```python
from build123d import *

# Parameters (mm, degrees)
SKETCH1_W                      = 229
SKETCH1_H                      = 200
BOSS_EXTRUDE1_DEPTH            = 1
CUT_EXTRUDE1_DEPTH             = 2
FILLET1_R                      = 8
FILLET2_R                      = 10
M3_CLEARANCE_HOLE1_AT_2_COUNT  = 2
M3_CLEARANCE_HOLE1_AT_2_PITCH  = 20
M3_CLEARANCE_HOLE1_AT_3_COUNT  = 2
M3_CLEARANCE_HOLE1_AT_3_PITCH  = 40
M3_CLEARANCE_HOLE1_AT_4_COUNT  = 2
M3_CLEARANCE_HOLE1_AT_4_PITCH  = 60
M3_CLEARANCE_HOLE1_AT_5_COUNT  = 2
M3_CLEARANCE_HOLE1_AT_5_PITCH  = 80
M3_CLEARANCE_HOLE1_AT_6_COUNT  = 2
M3_CLEARANCE_HOLE1_AT_6_PITCH  = 100
M3_CLEARANCE_HOLE1_AT_7_COUNT  = 2
M3_CLEARANCE_HOLE1_AT_7_PITCH  = 120
M3_CLEARANCE_HOLE1_AT_8_COUNT  = 2
M3_CLEARANCE_HOLE1_AT_8_PITCH  = 140
M3_CLEARANCE_HOLE1_AT_9_COUNT  = 2
M3_CLEARANCE_HOLE1_AT_9_PITCH  = 160
M3_CLEARANCE_HOLE1_AT_10_COUNT = 2
M3_CLEARANCE_HOLE1_AT_10_PITCH = 180
M3_CLEARANCE_HOLE2_AT_2_COUNT  = 2
M3_CLEARANCE_HOLE2_AT_2_PITCH  = 20
M3_CLEARANCE_HOLE2_AT_3_COUNT  = 2
M3_CLEARANCE_HOLE2_AT_3_PITCH  = 40
M3_CLEARANCE_HOLE2_AT_4_COUNT  = 2
M3_CLEARANCE_HOLE2_AT_4_PITCH  = 60
M3_CLEARANCE_HOLE2_AT_5_COUNT  = 2
M3_CLEARANCE_HOLE2_AT_5_PITCH  = 80
M3_CLEARANCE_HOLE2_AT_6_COUNT  = 2
M3_CLEARANCE_HOLE2_AT_6_PITCH  = 100
M3_CLEARANCE_HOLE2_AT_7_COUNT  = 2
M3_CLEARANCE_HOLE2_AT_7_PITCH  = 120
M3_CLEARANCE_HOLE2_AT_8_COUNT  = 2
M3_CLEARANCE_HOLE2_AT_8_PITCH  = 140
M3_CLEARANCE_HOLE2_AT_9_COUNT  = 2
M3_CLEARANCE_HOLE2_AT_9_PITCH  = 160
M3_CLEARANCE_HOLE2_AT_10_COUNT = 2
M3_CLEARANCE_HOLE2_AT_10_PITCH = 180
M3_CLEARANCE_HOLE2_AT_11_COUNT = 2
M3_CLEARANCE_HOLE2_AT_11_PITCH = 254.558441227
M3_CLEARANCE_HOLE2_AT_12_COUNT = 2
M3_CLEARANCE_HOLE2_AT_12_PITCH = 240.831891576
M3_CLEARANCE_HOLE2_AT_13_COUNT = 2
M3_CLEARANCE_HOLE2_AT_13_PITCH = 228.03508502
M3_CLEARANCE_HOLE2_AT_14_COUNT = 2
M3_CLEARANCE_HOLE2_AT_14_PITCH = 216.333076528
M3_CLEARANCE_HOLE2_AT_15_COUNT = 2
M3_CLEARANCE_HOLE2_AT_15_PITCH = 205.91260282
M3_CLEARANCE_HOLE2_AT_16_COUNT = 2
M3_CLEARANCE_HOLE2_AT_16_PITCH = 196.977156036
M3_CLEARANCE_HOLE2_AT_17_COUNT = 2
M3_CLEARANCE_HOLE2_AT_17_PITCH = 189.73665961
M3_CLEARANCE_HOLE2_AT_18_COUNT = 2
M3_CLEARANCE_HOLE2_AT_18_PITCH = 184.390889146
M3_CLEARANCE_HOLE2_AT_19_COUNT = 2
M3_CLEARANCE_HOLE2_AT_19_PITCH = 181.107702763
M3_CLEARANCE_HOLE2_AT_20_COUNT = 2
M3_CLEARANCE_HOLE2_AT_20_PITCH = 180
SKETCH7_R                      = 25
CUT_EXTRUDE2_DEPTH             = 10
FILLET3_R                      = 10
M4_CLEARANCE_HOLE1_AT_2_COUNT  = 2
M4_CLEARANCE_HOLE1_AT_2_PITCH  = 105
M4_CLEARANCE_HOLE1_AT_3_COUNT  = 2
M4_CLEARANCE_HOLE1_AT_3_PITCH  = 105
M4_CLEARANCE_HOLE1_AT_4_COUNT  = 2
M4_CLEARANCE_HOLE1_AT_4_PITCH  = 148.492424049
SKETCH10_R                     = 60
CUT_EXTRUDE3_DEPTH             = 10


with BuildPart() as part:
    # Sketch1 → Boss-Extrude1 (new body)
    with BuildSketch(Plane(origin=(0, 0, 0), x_dir=(1, 0, 0), z_dir=(0, 1, 0))):
        Rectangle(SKETCH1_W, SKETCH1_H)
    extrude(amount=BOSS_EXTRUDE1_DEPTH)

    # Sketch2 → Cut-Extrude1 (cut, through all)
    with BuildSketch(Plane(origin=(0, 1, 0), x_dir=(1, 0, 0), z_dir=(0, 1, 0))):
        Polygon((114.5, 60), (101.5, 73), (101.5, 100), (114.5, 100), align=None)
        Polygon((101.5, -100), (114.5, -100), (114.5, -60), (101.5, -73), align=None)
    extrude(amount=-CUT_EXTRUDE1_DEPTH, mode=Mode.SUBTRACT)

    # Fillet1
    fillet1_edges = [part.edges().sort_by_distance(p)[0] for p in [
        (114.5, 0.5, -60),
        (101.5, 0.5, -73),
        (101.5, 0.5, 73),
        (114.5, 0.5, 60),
    ]]
    fillet(fillet1_edges, radius=FILLET1_R)

    # Fillet2
    fillet2_edges = [part.edges().sort_by_distance(p)[0] for p in [
        (101.5, 0.5, -100),
        (101.5, 0.5, 100),
        (-114.5, 0.5, 100),
        (-114.5, 0.5, -100),
    ]]
    fillet(fillet2_edges, radius=FILLET2_R)

    # Sketch4 → M3 Clearance Hole1 (revolve, cut)
    with BuildSketch(Plane(origin=(-104.5, 0, -90), x_dir=(0, 0, -1), z_dir=(1, 0, 0))):
        Polygon((0, 0), (0, 1), (1.7, 1), (1.7, 0.025), (1.725, 0), align=None)
    m3_clearance_hole1 = revolve(axis=Axis((-104.5, -6.35, -90), (0, 1, 0)), mode=Mode.SUBTRACT)

    # M3 Clearance Hole1 at 2: M3 Clearance Hole1 ×2
    with Locations(*[(0, 0, i * M3_CLEARANCE_HOLE1_AT_2_PITCH) for i in range(1, M3_CLEARANCE_HOLE1_AT_2_COUNT)]):
        add(m3_clearance_hole1, mode=Mode.SUBTRACT)

    # M3 Clearance Hole1 at 3: M3 Clearance Hole1 ×2
    with Locations(*[(0, 0, i * M3_CLEARANCE_HOLE1_AT_3_PITCH) for i in range(1, M3_CLEARANCE_HOLE1_AT_3_COUNT)]):
        add(m3_clearance_hole1, mode=Mode.SUBTRACT)

    # M3 Clearance Hole1 at 4: M3 Clearance Hole1 ×2
    with Locations(*[(0, 0, i * M3_CLEARANCE_HOLE1_AT_4_PITCH) for i in range(1, M3_CLEARANCE_HOLE1_AT_4_COUNT)]):
        add(m3_clearance_hole1, mode=Mode.SUBTRACT)

    # M3 Clearance Hole1 at 5: M3 Clearance Hole1 ×2
    with Locations(*[(0, 0, i * M3_CLEARANCE_HOLE1_AT_5_PITCH) for i in range(1, M3_CLEARANCE_HOLE1_AT_5_COUNT)]):
        add(m3_clearance_hole1, mode=Mode.SUBTRACT)

    # M3 Clearance Hole1 at 6: M3 Clearance Hole1 ×2
    with Locations(*[(0, 0, i * M3_CLEARANCE_HOLE1_AT_6_PITCH) for i in range(1, M3_CLEARANCE_HOLE1_AT_6_COUNT)]):
        add(m3_clearance_hole1, mode=Mode.SUBTRACT)

    # M3 Clearance Hole1 at 7: M3 Clearance Hole1 ×2
    with Locations(*[(0, 0, i * M3_CLEARANCE_HOLE1_AT_7_PITCH) for i in range(1, M3_CLEARANCE_HOLE1_AT_7_COUNT)]):
        add(m3_clearance_hole1, mode=Mode.SUBTRACT)

    # M3 Clearance Hole1 at 8: M3 Clearance Hole1 ×2
    with Locations(*[(0, 0, i * M3_CLEARANCE_HOLE1_AT_8_PITCH) for i in range(1, M3_CLEARANCE_HOLE1_AT_8_COUNT)]):
        add(m3_clearance_hole1, mode=Mode.SUBTRACT)

    # M3 Clearance Hole1 at 9: M3 Clearance Hole1 ×2
    with Locations(*[(0, 0, i * M3_CLEARANCE_HOLE1_AT_9_PITCH) for i in range(1, M3_CLEARANCE_HOLE1_AT_9_COUNT)]):
        add(m3_clearance_hole1, mode=Mode.SUBTRACT)

    # M3 Clearance Hole1 at 10: M3 Clearance Hole1 ×2
    with Locations(*[(0, 0, i * M3_CLEARANCE_HOLE1_AT_10_PITCH) for i in range(1, M3_CLEARANCE_HOLE1_AT_10_COUNT)]):
        add(m3_clearance_hole1, mode=Mode.SUBTRACT)

    # Sketch6 → M3 Clearance Hole2 (revolve, cut)
    with BuildSketch(Plane(origin=(90.5, 0, -90), x_dir=(0, 0, -1), z_dir=(1, 0, 0))):
        Polygon((0, 0), (0, 1), (1.7, 1), (1.7, 0.025), (1.725, 0), align=None)
    m3_clearance_hole2 = revolve(axis=Axis((90.5, -6.35, -90), (0, 1, 0)), mode=Mode.SUBTRACT)

    # M3 Clearance Hole2 at 2: M3 Clearance Hole2 ×2
    with Locations(*[(-i * M3_CLEARANCE_HOLE2_AT_2_PITCH, 0, 0) for i in range(1, M3_CLEARANCE_HOLE2_AT_2_COUNT)]):
        add(m3_clearance_hole2, mode=Mode.SUBTRACT)

    # M3 Clearance Hole2 at 3: M3 Clearance Hole2 ×2
    with Locations(*[(-i * M3_CLEARANCE_HOLE2_AT_3_PITCH, 0, 0) for i in range(1, M3_CLEARANCE_HOLE2_AT_3_COUNT)]):
        add(m3_clearance_hole2, mode=Mode.SUBTRACT)

    # M3 Clearance Hole2 at 4: M3 Clearance Hole2 ×2
    with Locations(*[(-i * M3_CLEARANCE_HOLE2_AT_4_PITCH, 0, 0) for i in range(1, M3_CLEARANCE_HOLE2_AT_4_COUNT)]):
        add(m3_clearance_hole2, mode=Mode.SUBTRACT)

    # M3 Clearance Hole2 at 5: M3 Clearance Hole2 ×2
    with Locations(*[(-i * M3_CLEARANCE_HOLE2_AT_5_PITCH, 0, 0) for i in range(1, M3_CLEARANCE_HOLE2_AT_5_COUNT)]):
        add(m3_clearance_hole2, mode=Mode.SUBTRACT)

    # M3 Clearance Hole2 at 6: M3 Clearance Hole2 ×2
    with Locations(*[(-i * M3_CLEARANCE_HOLE2_AT_6_PITCH, 0, 0) for i in range(1, M3_CLEARANCE_HOLE2_AT_6_COUNT)]):
        add(m3_clearance_hole2, mode=Mode.SUBTRACT)

    # M3 Clearance Hole2 at 7: M3 Clearance Hole2 ×2
    with Locations(*[(-i * M3_CLEARANCE_HOLE2_AT_7_PITCH, 0, 0) for i in range(1, M3_CLEARANCE_HOLE2_AT_7_COUNT)]):
        add(m3_clearance_hole2, mode=Mode.SUBTRACT)

    # M3 Clearance Hole2 at 8: M3 Clearance Hole2 ×2
    with Locations(*[(-i * M3_CLEARANCE_HOLE2_AT_8_PITCH, 0, 0) for i in range(1, M3_CLEARANCE_HOLE2_AT_8_COUNT)]):
        add(m3_clearance_hole2, mode=Mode.SUBTRACT)

    # M3 Clearance Hole2 at 9: M3 Clearance Hole2 ×2
    with Locations(*[(-i * M3_CLEARANCE_HOLE2_AT_9_PITCH, 0, 0) for i in range(1, M3_CLEARANCE_HOLE2_AT_9_COUNT)]):
        add(m3_clearance_hole2, mode=Mode.SUBTRACT)

    # M3 Clearance Hole2 at 10: M3 Clearance Hole2 ×2
    with Locations(*[(-i * M3_CLEARANCE_HOLE2_AT_10_PITCH, 0, 0) for i in range(1, M3_CLEARANCE_HOLE2_AT_10_COUNT)]):
        add(m3_clearance_hole2, mode=Mode.SUBTRACT)

    # M3 Clearance Hole2 at 11: M3 Clearance Hole2 ×2
    with Locations(*[Vector(-0.707106781, 0, 0.707106781) * (i * M3_CLEARANCE_HOLE2_AT_11_PITCH) for i in range(1, M3_CLEARANCE_HOLE2_AT_11_COUNT)]):
        add(m3_clearance_hole2, mode=Mode.SUBTRACT)

    # M3 Clearance Hole2 at 12: M3 Clearance Hole2 ×2
    with Locations(*[Vector(-0.664363839, 0, 0.747409319) * (i * M3_CLEARANCE_HOLE2_AT_12_PITCH) for i in range(1, M3_CLEARANCE_HOLE2_AT_12_COUNT)]):
        add(m3_clearance_hole2, mode=Mode.SUBTRACT)

    # M3 Clearance Hole2 at 13: M3 Clearance Hole2 ×2
    with Locations(*[Vector(-0.613940614, 0, 0.789352217) * (i * M3_CLEARANCE_HOLE2_AT_13_PITCH) for i in range(1, M3_CLEARANCE_HOLE2_AT_13_COUNT)]):
        add(m3_clearance_hole2, mode=Mode.SUBTRACT)

    # M3 Clearance Hole2 at 14: M3 Clearance Hole2 ×2
    with Locations(*[Vector(-0.554700196, 0, 0.832050294) * (i * M3_CLEARANCE_HOLE2_AT_14_PITCH) for i in range(1, M3_CLEARANCE_HOLE2_AT_14_COUNT)]):
        add(m3_clearance_hole2, mode=Mode.SUBTRACT)

    # M3 Clearance Hole2 at 15: M3 Clearance Hole2 ×2
    with Locations(*[Vector(-0.485642931, 0, 0.874157276) * (i * M3_CLEARANCE_HOLE2_AT_15_PITCH) for i in range(1, M3_CLEARANCE_HOLE2_AT_15_COUNT)]):
        add(m3_clearance_hole2, mode=Mode.SUBTRACT)

    # M3 Clearance Hole2 at 16: M3 Clearance Hole2 ×2
    with Locations(*[Vector(-0.406138466, 0, 0.913811549) * (i * M3_CLEARANCE_HOLE2_AT_16_PITCH) for i in range(1, M3_CLEARANCE_HOLE2_AT_16_COUNT)]):
        add(m3_clearance_hole2, mode=Mode.SUBTRACT)

    # M3 Clearance Hole2 at 17: M3 Clearance Hole2 ×2
    with Locations(*[Vector(-0.316227766, 0, 0.948683298) * (i * M3_CLEARANCE_HOLE2_AT_17_PITCH) for i in range(1, M3_CLEARANCE_HOLE2_AT_17_COUNT)]):
        add(m3_clearance_hole2, mode=Mode.SUBTRACT)

    # M3 Clearance Hole2 at 18: M3 Clearance Hole2 ×2
    with Locations(*[Vector(-0.216930458, 0, 0.97618706) * (i * M3_CLEARANCE_HOLE2_AT_18_PITCH) for i in range(1, M3_CLEARANCE_HOLE2_AT_18_COUNT)]):
        add(m3_clearance_hole2, mode=Mode.SUBTRACT)

    # M3 Clearance Hole2 at 19: M3 Clearance Hole2 ×2
    with Locations(*[Vector(-0.110431526, 0, 0.993883735) * (i * M3_CLEARANCE_HOLE2_AT_19_PITCH) for i in range(1, M3_CLEARANCE_HOLE2_AT_19_COUNT)]):
        add(m3_clearance_hole2, mode=Mode.SUBTRACT)

    # M3 Clearance Hole2 at 20: M3 Clearance Hole2 ×2
    with Locations(*[(0, 0, i * M3_CLEARANCE_HOLE2_AT_20_PITCH) for i in range(1, M3_CLEARANCE_HOLE2_AT_20_COUNT)]):
        add(m3_clearance_hole2, mode=Mode.SUBTRACT)

    # Sketch7 → Cut-Extrude2 (cut)
    with BuildSketch(Plane(origin=(0, 0, 0), x_dir=(-1, 0, 0), z_dir=(0, -1, 0))):
        with Locations((-130.5, 0)):
            Circle(SKETCH7_R)
    extrude(amount=-CUT_EXTRUDE2_DEPTH, mode=Mode.SUBTRACT)

    # Fillet3
    fillet3_edges = [part.edges().sort_by_distance(p)[0] for p in [
        (114.5, 0.5, -19.209372712),
        (114.5, 0.5, 19.209372712),
    ]]
    fillet(fillet3_edges, radius=FILLET3_R)

    # Sketch9 → M4 Clearance Hole1 (revolve, cut)
    with BuildSketch(Plane(origin=(52.5, 1, -37.5), x_dir=(0, 0, 1), z_dir=(1, 0, 0))):
        Polygon((0, 0), (0, 1), (2.25, 1), (2.25, 0.025), (2.275, 0), align=None)
    m4_clearance_hole1 = revolve(axis=Axis((52.5, 7.35, -37.5), (0, -1, 0)), mode=Mode.SUBTRACT)

    # M4 Clearance Hole1 at 2: M4 Clearance Hole1 ×2
    with Locations(*[(0, 0, i * M4_CLEARANCE_HOLE1_AT_2_PITCH) for i in range(1, M4_CLEARANCE_HOLE1_AT_2_COUNT)]):
        add(m4_clearance_hole1, mode=Mode.SUBTRACT)

    # M4 Clearance Hole1 at 3: M4 Clearance Hole1 ×2
    with Locations(*[(-i * M4_CLEARANCE_HOLE1_AT_3_PITCH, 0, 0) for i in range(1, M4_CLEARANCE_HOLE1_AT_3_COUNT)]):
        add(m4_clearance_hole1, mode=Mode.SUBTRACT)

    # M4 Clearance Hole1 at 4: M4 Clearance Hole1 ×2
    with Locations(*[Vector(-0.707106781, 0, 0.707106781) * (i * M4_CLEARANCE_HOLE1_AT_4_PITCH) for i in range(1, M4_CLEARANCE_HOLE1_AT_4_COUNT)]):
        add(m4_clearance_hole1, mode=Mode.SUBTRACT)

    # Sketch10 → Cut-Extrude3 (cut)
    with BuildSketch(Plane(origin=(0, 1, 0), x_dir=(1, 0, 0), z_dir=(0, 1, 0))):
        with Locations((0, -15)):
            Circle(SKETCH10_R)
    extrude(amount=-CUT_EXTRUDE3_DEPTH, mode=Mode.SUBTRACT)


solid = part.part
```
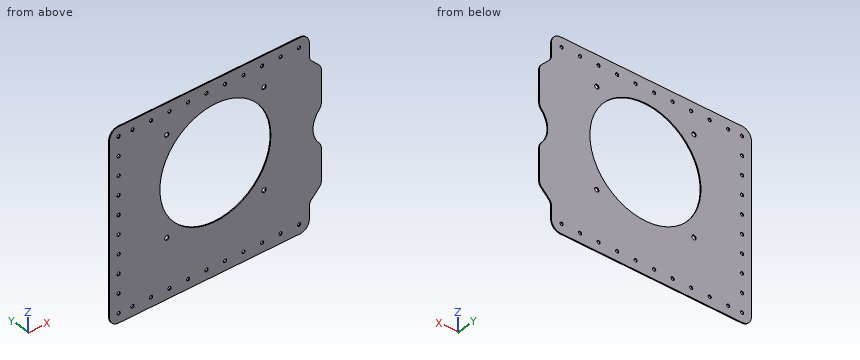
Build history of the part. All positions in model axes, mm. Coordinates: 2 decimals unless noted, no trailing zeros. Order: outer loops, then holes, each group sorted by start corner. A loop starts at its lowest first (then second) coordinate and runs counter-clockwise, first axis right, second up. Notation, with made-up numbers: (50, -22) -> (107, -22) arc R32 cw to (107, 5) -> close; hole circle Ø3 at (47, 11.5). An arc over 180 degrees is marked (long way). Answer in a Markdown table with one row per item. Add a question column.
Q1. Band-saw the part on A-A, the plane x = 18. List the corners of the cut face in (y, z).
Q2. Wall check: line 1 along Z through (x, y) = (-1.5, 0.8); line 2 along X through (y, z) = (0.6, 67.5); line 3 along X through (y, z) = (0.35, -37.5). Give the ranges that are in metal, low to high. Write a range as [from, to].
Q3. Band-saw the part on C-C, the plane y = 0.7. Give the number of separate pieces and of enclosed holes in the cut face, then the cut area to 3 significant figures.
Q4. Band-saw the part on B-B, the plane x = 41. List the corners of the cut face in (y, z), then the cut area to 3 significant figures.
Q5. Drop a flat-ended pin along its axis: pin 1 (8 mm diameter, centred on x = 41, z = -77.5, fed in from -Y). Give the stop position or say it passes through.
Answers follow:
| question | item | result |
|---|---|---|
| 1 | outline | (0, -100) -> (1, -100) -> (1, -42.24) -> (0, -42.24) -> close; (0, 72.24) -> (1, 72.24) -> (1, 100) -> (0, 100) -> close |
| 2 | line 1 | [-100, -44.98], [74.98, 100] |
| 2 | line 2 | [-114.5, -54.75], [-50.25, -29.05], [29.05, 50.25], [54.75, 107] |
| 2 | line 3 | [-114.5, -54.75], [-50.25, -29.05], [29.05, 50.25], [54.75, 114.5] |
| 3 | separate pieces | 1 |
| 3 | enclosed holes | 35 |
| 3 | area | 33,000 mm^2 |
| 4 | outline | (0, -100) -> (1, -100) -> (1, -28.81) -> (0, -28.81) -> close; (0, 58.81) -> (1, 58.81) -> (1, 100) -> (0, 100) -> close |
| 4 | area | 112 mm^2 |
| 5 | pin 1 | y = 0 |
